from build123d import *

# Parameters (mm, degrees)
SKETCH1_R           = 2
SKETCH1_R_2         = 1.5
SKETCH1_R_3         = 0.999995252
SKETCH1_W           = 2
SKETCH1_H           = 10
SKETCH1_W_2         = 6
SKETCH1_H_2         = 1
SKETCH1_W_3         = 10
SKETCH1_H_3         = 2
BOSS_EXTRUDE1_DEPTH = 2


with BuildPart() as part:
    # Sketch1 → Boss-Extrude1 (new body)
    with BuildSketch(Plane.XY):
        with BuildLine():
            Line((25, 2), (20, 2))
            Line((20, 2), (20, 0))
            Line((20, 0), (81, 0))
            Line((81, 0), (81, 2))
            Line((81, 2), (65, 2))
            ThreePointArc((65, 2), (66.199138226, 5.24860736), (69.221379911, 6.939003012))
            Line((69.221379911, 6.939003012), (160, 21.25))
            Line((160, 21.25), (204.582849115, 24.982568127))
            ThreePointArc((204.582849115, 24.982568127), (207.525828031, 24.315112137), (209.548736462, 22.075812274))
            ThreePointArc((209.548736462, 22.075812274), (219.060470979, 11.094065968), (233, 7))
            ThreePointArc((233, 7), (237.949747468, 4.949747468), (240, 0))
            Line((240, 0), (220, 0))
            Line((220, 0), (220, -2))
            Line((220, -2), (230, -2))
            ThreePointArc((230, -2), (231.885664581, -11.859196198), (237.276483238, -20.326696111))
            Line((237.276483238, -20.326696111), (247.82118659, -31.512397))
            ThreePointArc((247.82118659, -31.512397), (249.435371299, -34.047839158), (250, -37))
            Line((250, -37), (240, -37))
            Line((240, -37), (240, -41))
            ThreePointArc((240, -41), (239.707106781, -41.707106781), (239, -42))
            Line((239, -42), (231, -42))
            ThreePointArc((231, -42), (230.292893219, -41.707106781), (230, -41))
            Line((230, -41), (230, -37))
            Line((230, -37), (220.000007865, -37))
            Line((220.000007865, -37), (220.000007865, -39))
            Line((220.000007865, -39), (219.870131034, -39))
            ThreePointArc((219.870131034, -39), (217.168606934, -38.530057605), (214.784473011, -37.175441885))
            Line((214.784473011, -37.175441885), (200.000007865, -25))
            Line((200.000007865, -25), (160, -15))
            ThreePointArc((160, -15), (110, -7), (60, -15))
            ThreePointArc((60, -15), (40.396078054, -9.019609728), (20, -7))
            ThreePointArc((20, -7), (10.034517702, -5.41243098), (1.055638849, -0.806896552))
            ThreePointArc((1.055638849, -0.806896552), (0.646331624, 0), (1.055638849, 0.806896552))
            ThreePointArc((1.055638849, 0.806896552), (10.034517702, 5.41243098), (20, 7))
            ThreePointArc((20, 7), (23.535533906, 5.535533906), (25, 2))
        make_face()
        with Locations((10, 0)):
            Circle(SKETCH1_R, mode=Mode.SUBTRACT)
        with Locations((205, 20)):
            Circle(SKETCH1_R_2, mode=Mode.SUBTRACT)
        with Locations((110, -5.003081664)):
            Circle(SKETCH1_R_3, mode=Mode.SUBTRACT)
        with Locations((97, 5)):
            Circle(SKETCH1_R, mode=Mode.SUBTRACT)
        with Locations((205.2, -22.5)):
            Circle(SKETCH1_R, mode=Mode.SUBTRACT)
        with BuildLine():
            Line((66.32455532, -2), (100.63531967, -2))
            ThreePointArc((100.63531967, -2), (99.70444241, -4.376890478), (97.406972045, -5.489441931))
            ThreePointArc((97.406972045, -5.489441931), (83.509545549, -7.177146827), (69.809337188, -10.056574175))
            ThreePointArc((69.809337188, -10.056574175), (68.381496484, -6.545596578), (65.749595746, -3.818181818))
            ThreePointArc((65.749595746, -3.818181818), (65.371092731, -2.698488655), (66.32455532, -2))
        make_face(mode=Mode.SUBTRACT)
        with Locations((60, -7)):
            Rectangle(SKETCH1_W, SKETCH1_H, mode=Mode.SUBTRACT)
        with BuildLine():
            Line((17, -2), (53.67544468, -2))
            ThreePointArc((53.67544468, -2), (54.628907269, -2.698488655), (54.250404254, -3.818181818))
            ThreePointArc((54.250404254, -3.818181818), (51.797261355, -6.280290329), (50.33500013, -9.433333386))
            ThreePointArc((50.33500013, -9.433333386), (35.328622555, -6.114189089), (20, -5))
            ThreePointArc((20, -5), (17.878679656, -4.121320344), (17, -2))
        make_face(mode=Mode.SUBTRACT)
        with Locations((235, -39.5)):
            Rectangle(SKETCH1_W_2, SKETCH1_H_2, mode=Mode.SUBTRACT)
        with Locations((160, -7)):
            Rectangle(SKETCH1_W, SKETCH1_H, mode=Mode.SUBTRACT)
        with BuildLine():
            Line((170, -15.438446719), (195.626465602, -21.84506186))
            ThreePointArc((195.626465602, -21.84506186), (198.873506118, -21.75040587), (201.59533068, -19.977300424))
            Line((201.59533068, -19.977300424), (214.743385775, -4.964820224))
            ThreePointArc((214.743385775, -4.964820224), (215.570247155, -3.583733857), (215.858147077, -2))
            Line((215.858147077, -2), (166.32455532, -2))
            ThreePointArc((166.32455532, -2), (165.371092731, -2.698488655), (165.749595746, -3.818181818))
            ThreePointArc((165.749595746, -3.818181818), (168.874005788, -7.390008539), (170, -12))
            Line((170, -12), (170, -15.438446719))
        make_face(mode=Mode.SUBTRACT)
        with BuildLine():
            Line((119.36468033, -2), (153.67544468, -2))
            ThreePointArc((153.67544468, -2), (154.628907269, -2.698488655), (154.250404254, -3.818181818))
            ThreePointArc((154.250404254, -3.818181818), (151.618503516, -6.545596578), (150.190662812, -10.056574175))
            ThreePointArc((150.190662812, -10.056574175), (136.490454451, -7.177146827), (122.593027955, -5.489441931))
            ThreePointArc((122.593027955, -5.489441931), (120.29555759, -4.376890478), (119.36468033, -2))
        make_face(mode=Mode.SUBTRACT)
        with BuildLine():
            Line((225.879980597, -9.844071792), (220.058756659, -31.382600362))
            ThreePointArc((220.058756659, -31.382600362), (218.736154735, -32.766086526), (216.856615367, -32.404642783))
            Line((216.856615367, -32.404642783), (211.457170989, -27.95804153))
            ThreePointArc((211.457170989, -27.95804153), (210.382589597, -26.57746498), (210, -24.870320587))
            Line((210, -24.870320587), (210, -17.956008689))
            ThreePointArc((210, -17.956008689), (210.255911041, -16.54824526), (210.990898935, -15.320612934))
            Line((210.990898935, -15.320612934), (219.00942596, -6.165039937))
            ThreePointArc((219.00942596, -6.165039937), (223.906765634, -5.274169259), (225.879980597, -9.844071792))
        make_face(mode=Mode.SUBTRACT)
        with BuildLine():
            Line((155.22, 4), (158.067354896, 11.869573832))
            ThreePointArc((158.067354896, 11.869573832), (157.729169089, 13.823107559), (155.875224231, 14.525640207))
            Line((155.875224231, 14.525640207), (114.171743224, 7.95120241))
            ThreePointArc((114.171743224, 7.95120241), (111.753949876, 6.598885888), (110.794639295, 4))
            Line((110.794639295, 4), (155.22, 4))
        make_face(mode=Mode.SUBTRACT)
        with BuildLine():
            Line((162.73140024, 15.457687033), (196.499418938, 18.28481524))
            ThreePointArc((196.499418938, 18.28481524), (201.061804625, 16.721811294), (203, 12.305733488))
            Line((203, 12.305733488), (203, 4))
            Line((203, 4), (157.3468873, 4))
            Line((157.3468873, 4), (161.017577964, 14.145124952))
            ThreePointArc((161.017577964, 14.145124952), (161.682196092, 15.052484435), (162.73140024, 15.457687033))
        make_face(mode=Mode.SUBTRACT)
        with BuildLine():
            Line((206, 13.981517971), (206, 4))
            Line((206, 4), (223.586196304, 4))
            ThreePointArc((223.586196304, 4), (223.320669931, 4.852100267), (222.618096484, 5.402527076))
            ThreePointArc((222.618096484, 5.402527076), (215.414646092, 9.369582641), (209.598579041, 15.18341025))
            ThreePointArc((209.598579041, 15.18341025), (207.366422097, 15.878510075), (206, 13.981517971))
        make_face(mode=Mode.SUBTRACT)
        Polygon((166, 19.745335237), (175.965136254, 20.579637008), (176.131996608, 18.586609757), (166.166860354, 17.752307987), align=None, mode=Mode.SUBTRACT)
        Polygon((150.334018075, 17.701484711), (140.45601205, 16.144244533), (140.767460085, 14.168643328), (150.64546611, 15.725883506), align=None, mode=Mode.SUBTRACT)
        Polygon((121.011448036, 11.054162973), (120.7, 13.029764178), (130.578006025, 14.587004355), (130.88945406, 12.61140315), align=None, mode=Mode.SUBTRACT)
        Polygon((186.097132862, 19.420911528), (185.930272507, 21.413938779), (195.895408761, 22.24824055), (196.062269115, 20.255213299), align=None, mode=Mode.SUBTRACT)
        with BuildLine():
            Line((227.433137345, -19.428406141), (224.17644118, -31.47818195))
            ThreePointArc((224.17644118, -31.47818195), (224.519144651, -33.215805062), (226.107167967, -34))
            Line((226.107167967, -34), (243.359060381, -34))
            ThreePointArc((243.359060381, -34), (243.112035325, -32.708429631), (242.405829515, -31.599173688))
            Line((242.405829515, -31.599173688), (234.365889943, -23.070497611))
            ThreePointArc((234.365889943, -23.070497611), (232.608526335, -21.034670167), (231.035971848, -18.852929436))
            ThreePointArc((231.035971848, -18.852929436), (229.048405235, -17.975259461), (227.433137345, -19.428406141))
        make_face(mode=Mode.SUBTRACT)
        with Locations((140, 1)):
            Rectangle(SKETCH1_W_3, SKETCH1_H_3, mode=Mode.SUBTRACT)
        with Locations((160, 1)):
            Rectangle(SKETCH1_W_3, SKETCH1_H_3, mode=Mode.SUBTRACT)
        with Locations((180, 1)):
            Rectangle(SKETCH1_W_3, SKETCH1_H_3, mode=Mode.SUBTRACT)
        with Locations((200, 1)):
            Rectangle(SKETCH1_W_3, SKETCH1_H_3, mode=Mode.SUBTRACT)
    extrude(amount=BOSS_EXTRUDE1_DEPTH)


solid = part.part
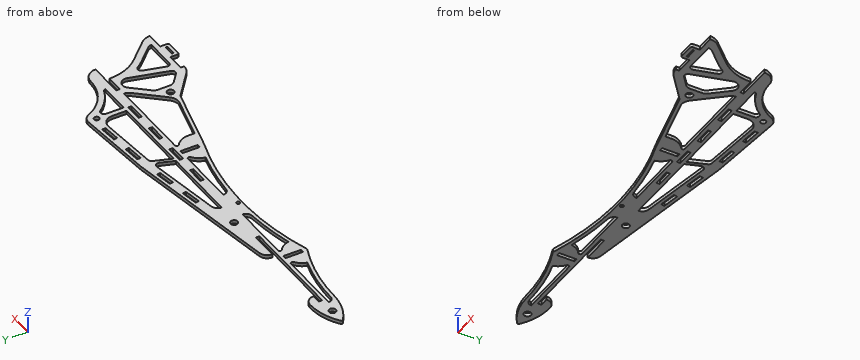
For this review, take the finished solid that the model builds, in its own axes (mm). Round coordinates to 2 decimals unless told otherwise and drop trailing zeros. Put each result on its own line as item: value. Start each with the question number.
1. Consider section A-A on z = 0.95. State how many separate pieces and enclosed holes the cut face has, plus the area to 3 significant figures.
2. For probe 1 along X at (y, z) = (3.5, 0.8); probe 2 along Y at (x, z) = (74, 1.6); probe 3 along Y at (x, z) = (141, 1.6), list the stretches that pass through material, from the lowest coordinate up. Write a range as [from, to].
3. Insertion check: P1, Ø1, axis at x = 180.5, z = 1, coming from the -Y side; P2, Ø1, axis at y = -14, z = 1.5, coming from the +X side; P3, Ø0.6, axis at x = 179.5, z = 0.5, coming from the +Y side. Each pin has a flat end and moves straight along its axis. Give the tip position at first contact, or say it passes through.
Result sheet:
1. separate pieces: 1
1. enclosed holes: 25
1. area: 3,510 mm^2
2. probe 1: [5.43, 24.77], [65.23, 95.68], [98.32, 239.06]
2. probe 2: [-11.1, -9.04], [-2, 0], [2, 7.69]
2. probe 3: [-10.03, -7.99], [-2, 0], [2, 4], [12.18, 14.21], [16.23, 18.25]
3. P1: y = -20.25
3. P2: x = 233.1
3. P3: y = 22.91
